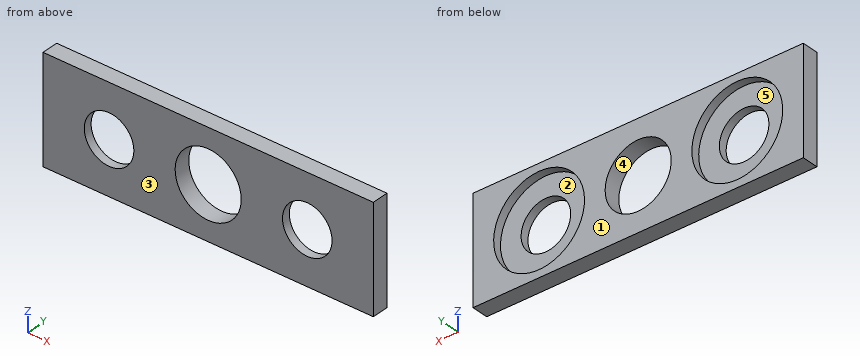
```python
from build123d import *

# Parameters (mm, degrees)
SKETCH1_W           = 63.5
SKETCH1_H           = 20.32
SKETCH1_R           = 4.7625
BOSS_EXTRUDE1_DEPTH = 3.175
SKETCH2_R           = 6.35
CUT_EXTRUDE1_DEPTH  = 6.35
SKETCH3_R           = 8.73125
CUT_EXTRUDE2_DEPTH  = 1.5875


with BuildPart() as part:
    # Sketch1 → Boss-Extrude1 (new body)
    with BuildSketch(Plane(origin=(0, 0, 0), x_dir=(1, 0, 0), z_dir=(0, 1, 0))):
        with Locations((31.75, 10.16)):
            Rectangle(SKETCH1_W, SKETCH1_H)
        with Locations(Location((12.7, 10.16, 0), (0, 0, 270))):
            Circle(SKETCH1_R, mode=Mode.SUBTRACT)
        with Locations(Location((50.8, 10.16, 0), (0, 0, 270))):
            Circle(SKETCH1_R, mode=Mode.SUBTRACT)
    extrude(amount=BOSS_EXTRUDE1_DEPTH)

    # Sketch2 → Cut-Extrude1 (cut)
    with BuildSketch(Plane(origin=(0, 3.175, 0), x_dir=(1, 0, 0), z_dir=(0, 1, 0))):
        with Locations(Location((31.75, 10.16, 0), (0, 0, 270))):
            Circle(SKETCH2_R)
    extrude(amount=-CUT_EXTRUDE1_DEPTH, mode=Mode.SUBTRACT)

    # Sketch3 → Cut-Extrude2 (cut)
    with BuildSketch(Plane(origin=(0, 3.175, 0), x_dir=(1, 0, 0), z_dir=(0, 1, 0))):
        with Locations(Location((12.7, 10.16, 0), (0, 0, 270))):
            Circle(SKETCH3_R)
        with Locations(Location((50.8, 10.16, 0), (0, 0, 270))):
            Circle(SKETCH3_R)
    extrude(amount=-CUT_EXTRUDE2_DEPTH, mode=Mode.SUBTRACT)


solid = part.part
```
Read the model definition and answer for the solid it produces. Units are mm, in the model's axes. Face numbers are marked on the shaded views. A direction names the side the tool comes from. Coordinates: 2 decimals unless noted, no trailing zeros. Loops run counter-clockwise (first coordinate to the right, second up) from the corner with the lowest first, then second, coordinate; pieces in that order, holes last.
(1) The part is cut by section A-A (z = -10.16). Determine the outline of the cut face in (x, y) (1 decimal).
Solution:
outline: (0, 0) - (7.9, 0) - (7.9, 1.6) - (4, 1.6) - (4, 3.2) - (0, 3.2) - close; (17.5, 0) - (25.4, 0) - (25.4, 3.2) - (21.4, 3.2) - (21.4, 1.6) - (17.5, 1.6) - close; (38.1, 0) - (46, 0) - (46, 1.6) - (42.1, 1.6) - (42.1, 3.2) - (38.1, 3.2) - close; (55.6, 0) - (63.5, 0) - (63.5, 3.2) - (59.5, 3.2) - (59.5, 1.6) - (55.6, 1.6) - close
(2) Consider line 1 along X through (y, z) = (2.1, -10.16); line 2 along X through (y, z) = (0.4, -10.16); line 3 along X through (y, z) = (2.75, -3.5). Determine where each line is inside the solid, lowest interval first.
Solution:
line 1: x = 0 to 3.97, 21.43 to 25.4, 38.1 to 42.07, 59.53 to 63.5
line 2: x = 0 to 7.94, 17.46 to 25.4, 38.1 to 46.04, 55.56 to 63.5
line 3: x = 0 to 7.05, 18.35 to 45.15, 56.45 to 63.5
(3) The part is cut by section B-B (x = 31.75). Determine the outline of the cut face in (y, z) (3 decimals), and give its area (3 significant figures).
Solution:
outline: (0, -20.32) - (3.175, -20.32) - (3.175, -16.51) - (0, -16.51) - close; (0, -3.81) - (3.175, -3.81) - (3.175, 0) - (0, 0) - close
area: 24.2 mm2
(4) Flat-ended cylindrical pins translate along their axes: pin 1 Ø5 at (x, z) = (30, -9.5) entering from +Y; pin 2 Ø8.5 at (x, z) = (14, -9.5) entering from +Y. Find the tip coordinate at first contact, or state that the pin passes through.
Solution:
pin 1: passes through
pin 2: stops at y = 1.59
(5) A tool of negligible diameter and unlimited length cuts with its end or side. For the marked faces 1 and 2, from which of +Z, -Z, +X, -X, +Y, -Y can it reach the whole face along a straight path? Write none if from no direction.
Solution:
face 1: +Z, -Z, +X, -X, +Y
face 2: +Y
(6) The part is cut by section D-D (x = 50.8). Determine the outline of the cut face in (y, z) (1 decimal).
Solution:
outline: (0, -20.3) - (3.2, -20.3) - (3.2, -18.9) - (1.6, -18.9) - (1.6, -14.9) - (0, -14.9) - close; (0, -5.4) - (1.6, -5.4) - (1.6, -1.4) - (3.2, -1.4) - (3.2, 0) - (0, 0) - close
(7) The part is cut by section C-C (y = 2.55). Determine the outline of the cut face in (x, z), and give its area (3 significant figures).
Solution:
outline: (0, -20.32) - (63.5, -20.32) - (63.5, 0) - (0, 0) - close; hole circle Ø17.46 at (12.7, -10.16); hole circle Ø12.7 at (31.75, -10.16); hole circle Ø17.46 at (50.8, -10.16)
area: 685 mm2
(8) The mould has two halves that part along X. Classify the marked faces 3, 4 and 5: released by +X, released by -X, zero draft, split by the parting line, or undercut.
Solution:
face 3: zero draft
face 4: undercut
face 5: undercut
